Autodesk Inventor part; units mm, degrees
ref_plane "YZ Plane" through (0, 0, 0) normal (1, 0, 0) x (0, 1, 0)
ref_plane "XZ Plane" through (0, 0, 0) normal (0, 1, 0) x (-1, 0, 0)
ref_plane "XY Plane" through (0, 0, 0) normal (0, 0, 1) x (1, 0, 0)
sketch "Sketch2" plane through (0, 0, 0) normal (0, 1, 0) x (-1, 0, 0)
  line L0 (0, 0) -> (38.5, 0)
  line L1 (38.5, 0) -> (38.5, -85.5)
  line L2 (38.5, -85.5) -> (0, -85.5)
  line L3 (0, -85.5) -> (0, 0)
  dimension "d5" = 38.5
  dimension "d6" = 85.5
extrude "Extrusion2" add sketch "Sketch2" along normal blind 4
sketch "Sketch4" plane through (0, 0, 0) normal (0, -1, 0) x (1, 0, 0)
  line L0 (0, 0) -> (4, 0)
  line L1 (4, 0) -> (4, -85.5)
  line L2 (4, -85.5) -> (0, -85.5)
  line L3 (0, -85.5) -> (0, 0)
  line L4 (-38.5, 0) -> (0, 0)
  line L5 (-38.5, 0) -> (-42.5, 0)
  line L6 (-42.5, 0) -> (-42.5, -85.5)
  line L7 (-42.5, -85.5) -> (-38.5, -85.5)
  line L8 (-38.5, -85.5) -> (-38.5, 0)
  line L9 (-42.5, -85.5) -> (4, -85.5)
  line L10 (4, -85.5) -> (4, -89.5)
  line L11 (4, -89.5) -> (-42.5, -89.5)
  line L12 (-42.5, -89.5) -> (-42.5, -85.5)
  line L13 (-42.5, 0) -> (4, 0)
  line L14 (4, 0) -> (4, 4)
  line L15 (4, 4) -> (-42.5, 4)
  line L16 (-42.5, 4) -> (-42.5, 0)
  dimension "d13" = 4
  dimension "d14" = 4
  dimension "d15" = 4
  dimension "d16" = 4
extrude "Extrusion3" add sketch "Sketch4" against normal blind 28 contours L4 L5 L16 L15 L14 L0 | L0 L1 L2 L3 | L2 L10 L11 L12 L7 L9 | L8 L7 L6 L5
fillet "Fillet1" radius 5 4 edges at (-42.5, 0, -42.75) (-19.25, 0, -89.5) (4, 0, -42.75) (-19.25, 0, 4)
fillet "Fillet2" radius 5 2 edges at (-41.0355, 1.4645, 2.5355) (-42.5, 16.5, 4)
fillet "Fillet3" radius 5 6 edges at (2.5355, 1.4645, 2.5355) (4, 16.5, 4) (2.5355, 1.4645, -88.0355) (4, 16.5, -89.5) (-41.0355, 1.4645, -88.0355) (-42.5, 16.5, -89.5)
sketch "Sketch5" plane through (0, 4, 0) normal (0, 1, 0) x (1, 0, 0)
  line L0 (0, 85.5) -> (0, 0)
  line L1 (0, 0) -> (-5.0038, 0)
  line L2 (0, 5.0038) -> (0, 0)
  line L3 (0, 85.5) -> (-5.0038, 85.5)
  line L4 (-5.0038, 85.5) -> (-5.0038, 80.4962)
  line L5 (-5.0038, 80.4962) -> (0, 80.4962)
  line L6 (0, 80.4962) -> (0, 85.5)
  circle A0 centre (-5.0038, 80.4962) radius 3
  line L7 (0, 85.5) -> (-38.5, 85.5)
  line L8 (-38.5, 85.5) -> (-33.4962, 85.5)
  line L9 (-33.4962, 85.5) -> (-33.4962, 80.4962)
  line L10 (-33.4962, 80.4962) -> (-38.5, 80.4962)
  line L11 (-38.5, 80.4962) -> (-38.5, 85.5)
  circle A1 centre (-33.4962, 80.4962) radius 3
  line L12 (0, 0) -> (-38.5, 0)
  line L13 (-38.5, 0) -> (-33.4962, 0)
  line L14 (-33.4962, 0) -> (-33.4962, 5.0038)
  line L15 (-33.4962, 5.0038) -> (-38.5, 5.0038)
  line L16 (-38.5, 5.0038) -> (-38.5, 0)
  circle A2 centre (-33.4962, 5.0038) radius 3
  dimension "d25" = 5.0038
  dimension "d26" = 5.0038
  dimension "d27" = 6
  dimension "d28" = 5.0038
  dimension "d29" = 5.0038
  dimension "d30" = 6
  dimension "d31" = 5.0038
  dimension "d32" = 5.0038
  dimension "d33" = 6
extrude "Extrusion4" add sketch "Sketch5" along normal blind 23 contours A0 L4 L5 | L5 L4 A0 | A1 L10 L9 | L9 L10 A1 | A2 L15 L14 | L14 L15 A2
sketch "Sketch6" plane through (-33.4962, 27, -5.0038) normal (0, 1, 0) x (1, 0, 0)
  circle A0 centre (0, 0) radius 1.5
  point P0 (33.4962, -5.0038)
  dimension "d36" = 3
sketch "Sketch7" plane through (-33.4962, 27, -80.4962) normal (0, 1, 0) x (1, 0, 0)
  circle A0 centre (0, 0) radius 3
  circle A1 centre (0, 0) radius 1.5
  point P0 (33.4962, -80.4962)
  dimension "d37" = 3
sketch "Sketch8" plane through (-5.0038, 27, -80.4962) normal (0, 1, 0) x (1, 0, 0)
  circle A0 centre (0, 0) radius 3
  circle A1 centre (0, 0) radius 1.5
  point P0 (5.0038, -80.4962)
  dimension "d38" = 3
extrude "Extrusion5" cut sketch "Sketch6" against normal blind 15
extrude "Extrusion6" cut sketch "Sketch7" against normal blind 15 contours A1
extrude "Extrusion7" cut sketch "Sketch8" against normal blind 15 contours A1
properties part number "Bottomcase"
Model file for the job. Use its own axes, mm. A direction names the side the tool comes from. Give positions to 0.01 mm unless a question says otherwise; leave off trailing zeros. Loops run counter-clockwise (first coordinate to the right, second up) from the corner with the lowest first, then second, coordinate; pieces in that order, holes last. Notation, with made-up numbers: (14, -28) - (53, -28) arc R25 ccw to (53, 0) - close; hole circle Ø1 at (52, 41). An arc over 180 degrees is marked (long way). One line per item, written item: value. Start each with the question number.
1. Slice it at A-A (z = -35.5). List the corners of the cut face in (x, y), plus the area to 3 significant figures.
2. Which spindle directions (+Z, -Z, +X, -X, +Y, -Y) get a long thin tool onto all of the face, cutting with end or side? Do faces 1 (the flat face through (-19, 16, 4)), 2 (the flat face through (-34, 12, -81)). Say none if no direction does.
3. Slice it at B-B (y = 24.5). List the corners of the cut face in (x, z), plus the area to 3 significant figures.
4. Probe L1, parallel to X at y = 19, z = -51; L2, parallel to Z at x = -17, y = 14; L3, parallel to Y at x = -30, z = -68. List the from-to ranges inside material, lowest first. Write a range as from..to.
5. Slice it at D-D (y = 9.25). List the corners of the cut face in (x, z).
6. Pin check, flat tips, straight feed: pin 1 (5 mm diameter, centred on x = -35, z = -79.5, fed in from +Y); pin 2 (3.5 mm diameter, centred on x = -33.5, z = -80.5, fed in from -Y); pin 3 (1.5 mm diameter, centred on x = -34, z = -80, fed in from +Y); pin 4 (3 mm diameter, centred on x = -34, z = -21.5, fed in from +Y). Stop position of each tip, or through.
7. Slice it at C-C (x = -14). List the corners of the cut face in (y, z), plus the area to 3 significant figures.
8. Pull direction Z, two halves, no side cores. Call faces 3 (the flat face through (0, 16, -43)), 4 (the cylindrical face through (3, 16, 2)), 5 (the cylindrical face through (-41.07, 16.34, -88)), 6 (the flat face through (-42.5, 16, -42)): pulls with the +Z half, pulls with the -Z half, needs draft (parallel to the pull), parting line crosses it, or undercut.
Solution:
1. outline: (-42.5, 5) arc R5 ccw to (-37.5, 0) - (-1, 0) arc R5 ccw to (4, 5) - (4, 28) - (0, 28) - (0, 4) - (-38.5, 4) - (-38.5, 28) - (-42.5, 28) - close
1. area: 367 mm^2
2. face 1: +Z, +X, -X, +Y, -Y
2. face 2: +Y
3. outline: (-42.5, -84.5) arc R5 ccw to (-37.5, -89.5) - (-1, -89.5) arc R5 ccw to (4, -84.5) - (4, -1) arc R5 ccw to (-1, 4) - (-37.5, 4) arc R5 ccw to (-42.5, -1) - close; circle Ø6 at (-33.5, -80.5); circle Ø6 at (-33.5, -5); circle Ø6 at (-5, -80.5); hole (-38.5, -85.5) - (0, -85.5) - (0, 0) - (-38.5, 0) - close; hole circle Ø3 at (-33.5, -80.5); hole circle Ø3 at (-33.5, -5); hole circle Ø3 at (-5, -80.5)
3. area: 1,100 mm^2
4. L1: x = -42.5..-38.5, 0..4
4. L2: z = -89.5..-85.5, 0..4
4. L3: y = 0..4
5. outline: (-42.5, -84.5) arc R5 ccw to (-37.5, -89.5) - (-1, -89.5) arc R5 ccw to (4, -84.5) - (4, -1) arc R5 ccw to (-1, 4) - (-37.5, 4) arc R5 ccw to (-42.5, -1) - close; circle Ø6 at (-33.5, -80.5); circle Ø6 at (-33.5, -5); circle Ø6 at (-5, -80.5); hole (-38.5, -85.5) - (0, -85.5) - (0, 0) - (-38.5, 0) - close
6. pin 1: stops at y = 27
6. pin 2: stops at y = 0
6. pin 3: stops at y = 12
6. pin 4: stops at y = 4
7. outline: (0, -84.5) arc R5 ccw to (5, -89.5) - (28, -89.5) - (28, -85.5) - (4, -85.5) - (4, 0) - (28, 0) - (28, 4) - (5, 4) arc R5 ccw to (0, -1) - close
7. area: 555 mm^2
8. face 3: undercut
8. face 4: pulls with the +Z half
8. face 5: pulls with the -Z half
8. face 6: needs draft
